The drawing under review shows one solid part. Ordinate dimensions are in mm from its lowest x, y, z. Coordinates: 2 decimals unless noted, no trailing zeros. Write each loop counter-clockwise with the first axis right and the second up, starting at its lowest first coordinate (ties: lowest second). Pieces come first, ordered by that corner, then holes.
Q1. Mouldability with a two-part tool opening along Y and no side actions: class the marked faces 1, 2, 3 and 4 as pulls with the +Y half, pulls with the -Y half, needs draft (parallel to the pull), parting line crosses it, or undercut.
Q2. Take a section at D-D (y = 45). Give the boundary of the cut face in (x, z).
Q3. Take a section at C-C (z = 4.75). Give the boundary of the cut face in (x, y) (3 decimals), and give its area (3 significant figures).
Q4. Take a section at A-A (x = 57.5). Give the boundary of the cut face in (y, z), and give its area (3 significant figures).
Q5. Take a section at B-B (y = 30). Give the boundary of the cut face in (x, z).
Q6. For probe 1 along Y at (x, z) = (12.5, 5.5); probe 2 along X at (y, z) = (45, 4.5); probe 3 along Y at (x, z) = (11.5, 7), list the stretches that pass through material, from the lowest coordinate up.
Q7. Insertion check: pin 1 (1.9 mm diameter, centred on x = 12.5, y = 15, fed in from +Z). The pin has a flat end and moves straight along its axis. Give the tip position at first contact, or say it passes through.
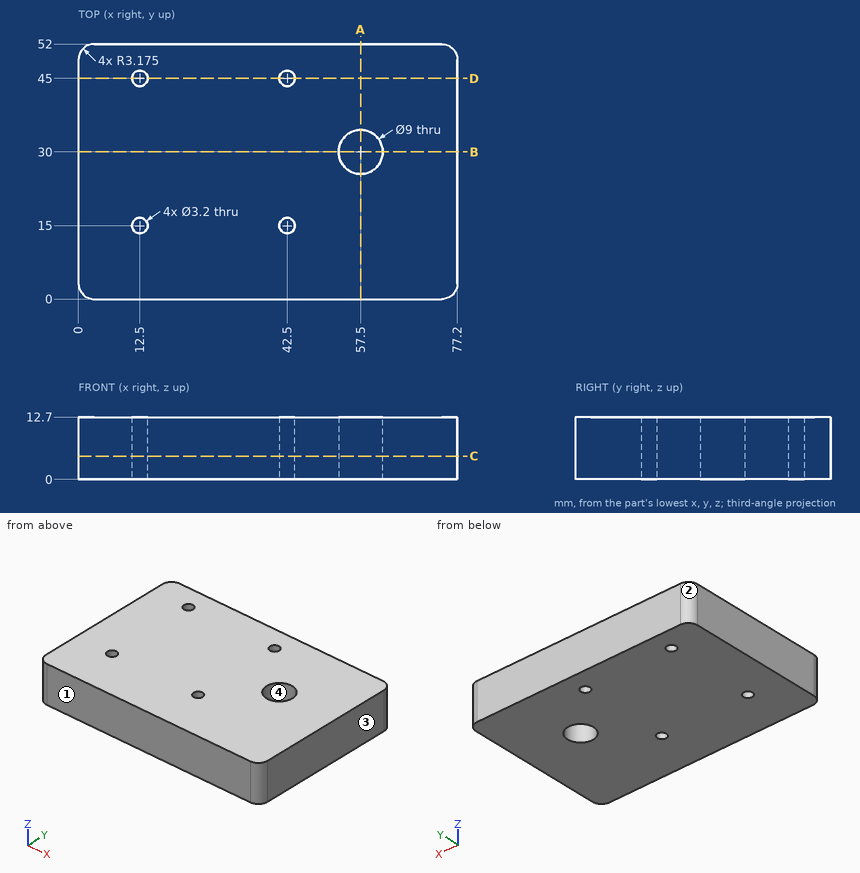
Response:
1. face 1: pulls with the -Y half
1. face 2: pulls with the +Y half
1. face 3: needs draft
1. face 4: undercut
2. outline: (0, 0) - (10.9, 0) - (10.9, 12.7) - (0, 12.7) - close; (14.1, 0) - (40.9, 0) - (40.9, 12.7) - (14.1, 12.7) - close; (44.1, 0) - (77.2, 0) - (77.2, 12.7) - (44.1, 12.7) - close
3. outline: (0, 3.175) arc R3.175 ccw to (3.175, 0) - (74.025, 0) arc R3.175 ccw to (77.2, 3.175) - (77.2, 48.825) arc R3.175 ccw to (74.025, 52) - (3.175, 52) arc R3.175 ccw to (0, 48.825) - close; hole circle Ø3.2 at (12.5, 15); hole circle Ø3.2 at (12.5, 45); hole circle Ø3.2 at (42.5, 15); hole circle Ø3.2 at (42.5, 45); hole circle Ø9 at (57.5, 30)
3. area: 3,910 mm2
4. outline: (0, 0) - (25.5, 0) - (25.5, 12.7) - (0, 12.7) - close; (34.5, 0) - (52, 0) - (52, 12.7) - (34.5, 12.7) - close
4. area: 546 mm2
5. outline: (0, 0) - (53, 0) - (53, 12.7) - (0, 12.7) - close; (62, 0) - (77.2, 0) - (77.2, 12.7) - (62, 12.7) - close
6. probe 1: y = 0 to 13.4, 16.6 to 43.4, 46.6 to 52
6. probe 2: x = 0 to 10.9, 14.1 to 40.9, 44.1 to 77.2
6. probe 3: y = 0 to 13.75, 16.25 to 43.75, 46.25 to 52
7. pin 1: passes through
